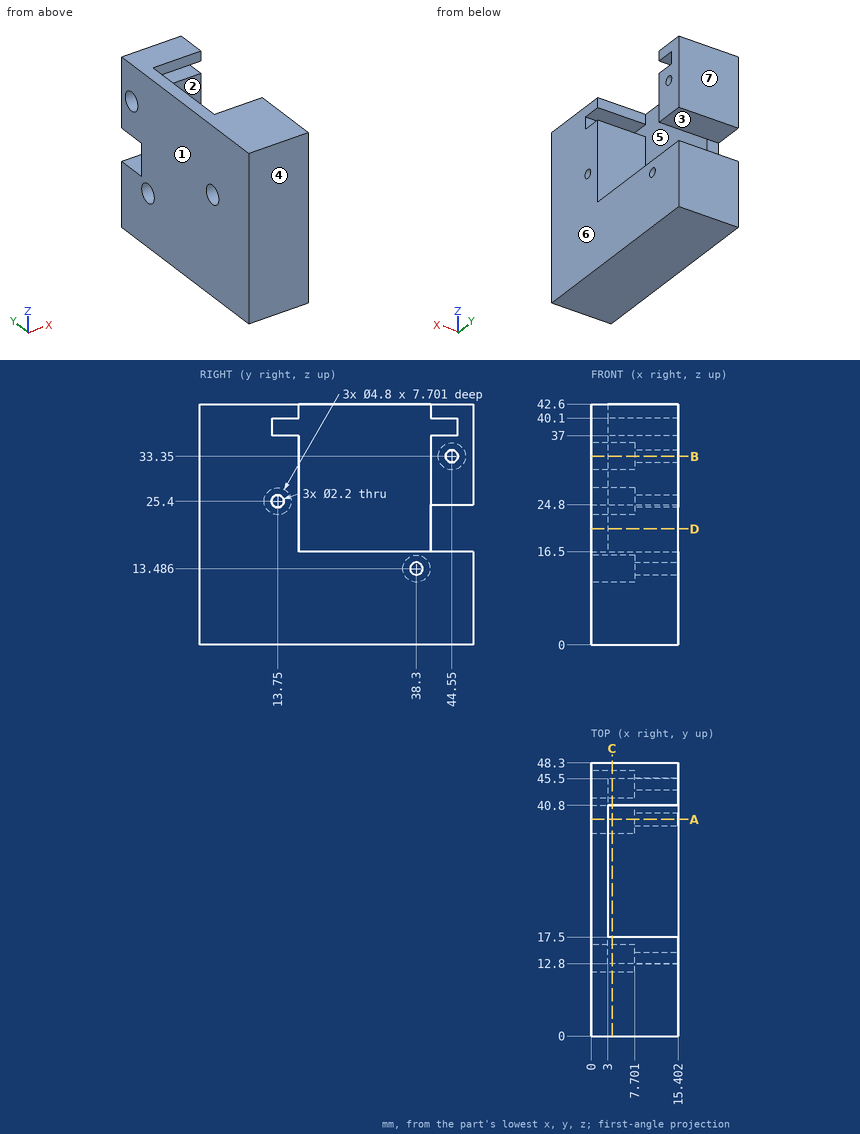
Part print with two shaded views. Sizes in mm from the minimum x, y, z corner. A direction names the side the tool comes from. Round coordinates to 2 decimals unless told otherwise and drop trailing zeros. Loops run counter-clockwise (first coordinate to the right, second up) from the corner with the lowest first, then second, coordinate; pieces in that order, holes last. Notation, with made-up numbers: (-22.75, 75) - (-8.75, 75) arc R20 ccw to (-8.75, 100) - close; hole circle Ø8 at (25, -21.5). An arc over 180 degrees is marked (long way). Put each result on its own line as item: value.
1. Slice it at C-C on x = 3.75. List the corners of the cut face in (y, z).
Geometry check:
outline: (0, 0) - (48.3, 0) - (48.3, 16.5) - (17.5, 16.5) - (17.5, 37) - (12.8, 37) - (12.8, 40.1) - (17.5, 40.1) - (17.5, 42.6) - (0, 42.6) - close; (40.8, 24.8) - (48.3, 24.8) - (48.3, 42.6) - (40.8, 42.6) - (40.8, 40.1) - (45.5, 40.1) - (45.5, 37) - (40.8, 37) - close; hole circle Ø4.8 at (13.75, 25.4); hole circle Ø4.8 at (38.3, 13.49); hole circle Ø4.8 at (44.55, 33.35)
2. Slice it at A-A on y = 38.3. List the corners of the cut face in (x, z).
Geometry check:
outline: (0, 0) - (15.4, 0) - (15.4, 12.39) - (7.7, 12.39) - (7.7, 11.09) - (0, 11.09) - close; (0, 15.89) - (7.7, 15.89) - (7.7, 14.59) - (15.4, 14.59) - (15.4, 16.5) - (3, 16.5) - (3, 42.6) - (0, 42.6) - close
3. Slice it at B-B on z = 33.35. List the corners of the cut face in (x, y).
Geometry check:
outline: (0, 0) - (15.4, 0) - (15.4, 17.5) - (3, 17.5) - (3, 40.8) - (15.4, 40.8) - (15.4, 43.45) - (7.7, 43.45) - (7.7, 42.15) - (0, 42.15) - close; (0, 46.95) - (7.7, 46.95) - (7.7, 45.65) - (15.4, 45.65) - (15.4, 48.3) - (0, 48.3) - close
4. Wall check: line 1 (Y direction, x = 9.75, z = 33.35); line 2 (Z direction, x = 10.5, y = 44.55); line 3 (Y direction, x = 13.75, z = 25.4). Give the ranges that are in metal, low to high.
Geometry check:
line 1: 0 to 17.5, 40.8 to 43.45, 45.65 to 48.3
line 2: 0 to 16.5, 24.8 to 32.25, 34.45 to 37, 40.1 to 42.6
line 3: 0 to 12.65, 14.85 to 17.5, 40.8 to 48.3
5. 3-axis set-ups, long thin cutter, end or side, ignore diameter. For the marked faces 1, 2 and 3: which of +Z, -Z, +X, -X, +Y, -Y reach the whole face in a straight line?
Geometry check:
face 1: +Z, -Z, -X, +Y, -Y
face 2: +Z, +X
face 3: +X, -X, +Y
6. Pin check, flat tips, straight feed: P1, Ø4.5, axis at y = 38.3, z = 13.49, coming from the -X side; P2, Ø2, axis at x = 4.5, z = 18.5, coming from the +Y side; P3, Ø1.3, axis at y = 38.3, z = 13.49, coming from the -X side; P4, Ø2.5, axis at x = 2, z = 20.5, coming from the +Y side. Stop position of each tip, or through.
Geometry check:
P1: x = 7.7
P2: y = 17.5
P3: through
P4: y = 40.8
7. Two-plate mould, pull along Y, no slides. Class the marked faces 4, 5, 6 and 7: released by +Y, released by -Y, zero draft, split by the parting line, or undercut.
Geometry check:
face 4: released by -Y
face 5: undercut
face 6: zero draft
face 7: released by +Y
8. Slice it at D-D on z = 20.5. List the corners of the cut face in (x, y).
Geometry check:
outline: (0, 0) - (15.4, 0) - (15.4, 17.5) - (3, 17.5) - (3, 40.8) - (0, 40.8) - close
